Work out the finished part from the listing and answer in its coordinate system (mm). Face numbers are marked on the shaded views. A direction names the side the tool comes from. Coordinates: 2 decimals unless noted, no trailing zeros. Order: outer loops, then holes, each group sorted by start corner. A loop starts at its lowest first (then second) coordinate and runs counter-clockwise, first axis right, second up. Notation, with made-up numbers: M 87,13.25 L 121,13.25 A9 cw 121,18.25 Z; hole C 70,18 d7. An arc over 180 degrees is marked long. Use a Markdown table: item, result.
from build123d import *

# Parameters (mm, degrees)
F0_R     = 17.775209
F1_DEPTH = 25.4


with BuildPart() as f1:
    # F0 (on Front) → F1 (new body)
    with BuildSketch(Plane.XZ):
        with BuildLine():
            ThreePointArc((-66.587123, -18.142906), (-42.667153, -6.543066), (-32.977377, 18.212327))
            ThreePointArc((-32.977377, 18.212327), (-42.667153, 42.96772), (-66.587123, 54.567559))
            ThreePointArc((-66.587123, 54.567559), (-105.912113, 18.212327), (-66.587123, -18.142906))
        make_face()
        with Locations((-69.444745, 18.212327)):
            Circle(F0_R, mode=Mode.SUBTRACT)
        with BuildLine():
            ThreePointArc((-66.587123, 54.567559), (-42.667153, 42.96772), (-32.977377, 18.212327))
            ThreePointArc((-32.977377, 18.212327), (-42.667153, -6.543066), (-66.587123, -18.142906))
            Line((-66.587123, -18.142906), (50.354917, -18.142906))
            Line((50.354917, -18.142906), (50.354917, 5.00767))
            Line((50.354917, 5.00767), (-17.176457, 5.00767))
            ThreePointArc((-17.176457, 5.00767), (-23.921096, 18.288839), (-16.882842, 31.41677))
            Line((-16.882842, 31.41677), (50.354917, 31.41677))
            Line((50.354917, 31.41677), (50.354917, 50.795339))
            ThreePointArc((50.354917, 50.795339), (45.72161, 53.463349), (40.490307, 54.567559))
            Line((40.490307, 54.567559), (-66.587123, 54.567559))
        make_face()
        with BuildLine():
            Line((50.354917, 54.567559), (40.490307, 54.567559))
            ThreePointArc((40.490307, 54.567559), (45.72161, 53.463349), (50.354917, 50.795339))
            Line((50.354917, 50.795339), (50.354917, 54.567559))
        make_face()
    extrude(amount=F1_DEPTH)


solid = f1.part
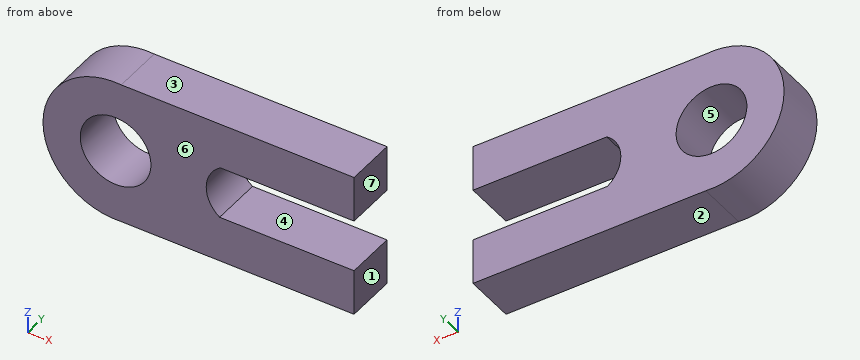
(1) A cutting plane is placed at A-A (x = -3). Determine the outline of the cut face in (y, z), then the cut area to 3 significant figures.
Conclusion:
| item | result |
|---|---|
| outline | M -25.4,-18.14 L 0,-18.14 L 0,5.01 L -25.4,5.01 Z; M -25.4,31.42 L 0,31.42 L 0,54.57 L -25.4,54.57 Z |
| area | 1,180 mm2 |
(2) Given P1, Ø3, axis at y = -6, z = 44.5, coming from the -X side; P2, Ø7.5, axis at x = 15.5, y = -7.5, coming from the +Z side; P3, Ø7.5, axis at x = 5, y = -17, coming from the -Z side, each flat-ended and moving along its own axis, determine where each tip first touches the part or whether it passes through.
Conclusion:
| item | result |
|---|---|
| P1 | x = -96.19 |
| P2 | z = 54.57 |
| P3 | z = -18.14 |
(3) Straight lines are drawn through the part: L1, parallel to Z at x = -15, y = -10.75; L2, parallel to Z at x = -24.5, y = -23.75; L3, parallel to X at y = -4, z = 10. For each, find the intervals that lie inside material, in ascending order.
Conclusion:
| item | result |
|---|---|
| L1 | -18.14 to 5.01, 31.42 to 54.57 |
| L2 | -18.14 to 54.57 |
| L3 | -104.98 to -85.21, -53.68 to -21.73 |
(4) A cutting plane is placed at B-B (z = 27). Determine the outline of the cut face in (x, y), then the cut area to 3 significant figures.
Conclusion:
| item | result |
|---|---|
| outline | M -104.84,-25.4 L -84.9,-25.4 L -84.9,0 L -104.84,0 Z; M -53.99,-25.4 L -21.24,-25.4 L -21.24,0 L -53.99,0 Z |
| area | 1,340 mm2 |
(5) A cutting plane is placed at D-D (z = -14). Determine the outline of the cut face in (x, y), then the cut area to 3 significant figures.
Conclusion:
| item | result |
|---|---|
| outline | M -86.54,-25.4 L 50.35,-25.4 L 50.35,0 L -86.54,0 Z |
| area | 3,480 mm2 |
(6) Which of the six approach directions +Z, -Z, +X, -X, +Y, -Y give full straight-line access (tool end or side, diameter ignored) to the marked faces 1, 2, 3 and 4?
Conclusion:
| item | result |
|---|---|
| face 1 | +Z, -Z, +X, +Y, -Y |
| face 2 | -Z, +X, +Y, -Y |
| face 3 | +Z, +X, +Y, -Y |
| face 4 | +X, +Y, -Y |
(7) Determine the mould class of the marked faces 5, 6 and 7 for opening direction X: pulls with the +X half, pulls with the -X half, needs draft (parallel to the pull), parting line crosses it, or undercut.
Conclusion:
| item | result |
|---|---|
| face 5 | undercut |
| face 6 | needs draft |
| face 7 | pulls with the +X half |
(8) A cutting plane is placed at C-C (y = -4.75). Determine the outline of the cut face in (x, z).
Conclusion:
| item | result |
|---|---|
| outline | M -66.59,-18.14 L 50.35,-18.14 L 50.35,5.01 L -17.18,5.01 A16.1 cw -16.88,31.42 L 50.35,31.42 L 50.35,54.57 L -66.59,54.57 A36.47 ccw long Z; hole C -69.44,18.21 d35.55 |
